Input: dimensioned drawing with shaded views. Units: mm. Origin: part minimum x, y, z. A direction names the side the tool comes from. Round coordinates to 2 decimals unless told otherwise and drop trailing zeros. Write each loop counter-clockwise with the first axis right and the second up, starting at its lowest first coordinate (ties: lowest second). Pieces come first, ordered by that corner, then holes. Notation, with made-up numbers: M -39.75,79.5 L 8.25,79.5 A31 ccw 8.25,106.5 Z; hole C 38,41.5 d10. An arc over 180 degrees is marked long. Put each result on its own line as item: value. Start each with the question number.
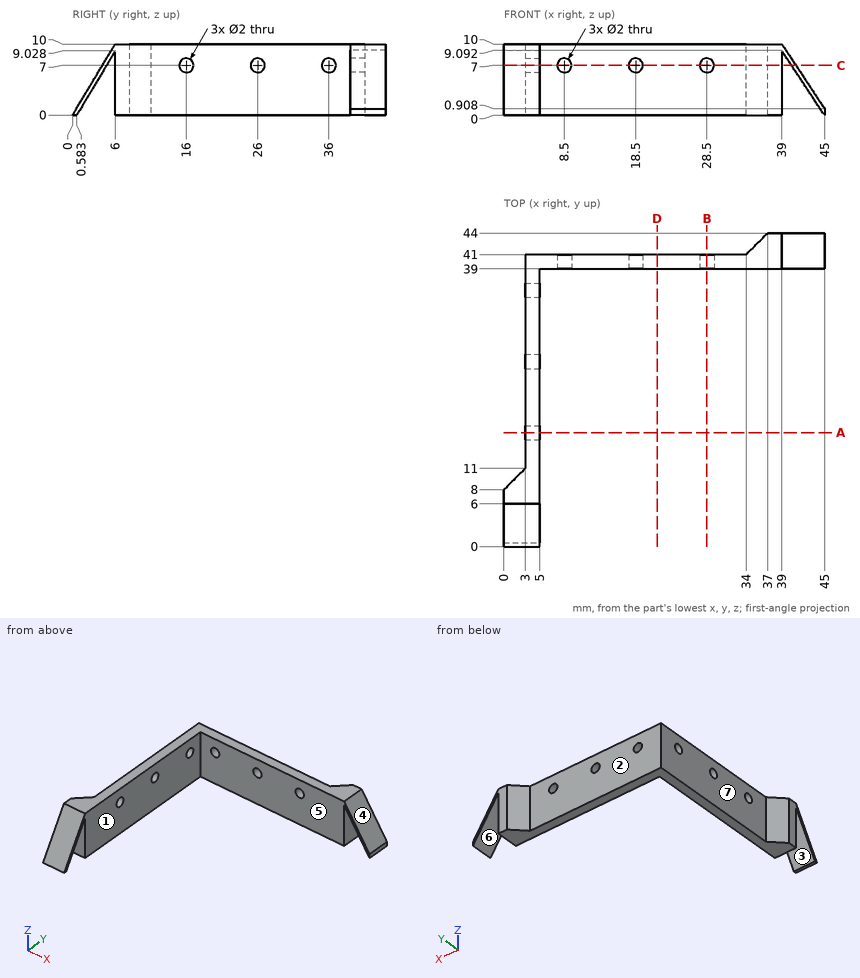
1) First-contact query: pin 1 (1.6 mm diameter, centred on x = 18.5, z = 7, fed in from +Y); pin 2 (3 mm diameter, centred on y = 27, z = 8.5, fed in from -X); pin 3 (1.5 mm diameter, centred on x = 23, z = 2.5, fed in from -Y); pin 4 (2.5 mm diameter, centred on y = 16, z = 7, fed in from +X). Flat tips, straight axial feed; report the tip coordinate or a pass-through.
2) Draft query along X for the marked faces 5, 6 and 7. Return one class per face: +X half, -X half, draft (parallel to the pull), parting line (faces both ways), or undercut.
3) Ray query, probe 1 along Z at (x, y) = (3.8, 16); probe 2 along Y at (x, z) = (14.5, 0.75); probe 3 along X at (y, z) = (8, 2.5). Return the intervals inside material, ascending.
4) Section A-A, the plane y = 16. Output: boundary loops of the cut face in (x, z), and give its area (3 significant figures).
5) Section D-D, the plane x = 21.5. Output: boundary loops of the cut face in (y, z), and give its area (3 significant figures).
6) Access query for the marked faces 1, 2, 3 and 4. Directions: +Z, -Z, +X, -X, +Y, -Y. A direction counts if a zero-diameter tool reaches every point of the face in a straight line with its end or side. Return the directions, or none.
7) Section B-B, the plane x = 28.5. Output: boundary loops of the cut face in (y, z), and give its area (3 significant figures).
8) Section C-C, the plane z = 7. Give the number of separate pieces and of enclosed holes in the cut face, and give its area (3 significant figures).
Solved:
1. pin 1: passes through
1. pin 2: stops at x = 3
1. pin 3: stops at y = 39
1. pin 4: stops at x = 5
2. face 5: draft
2. face 6: undercut
2. face 7: -X half
3. probe 1: z = 0 to 6, 8 to 10
3. probe 2: y = 39 to 41
3. probe 3: x = 0 to 5
4. outline: M 3,0 L 5,0 L 5,6 L 3,6 Z; M 3,8 L 5,8 L 5,10 L 3,10 Z
4. area: 16.0 mm2
5. outline: M 39,0 L 41,0 L 41,10 L 39,10 Z
5. area: 20.0 mm2
6. face 1: +Z, -Z, +X, -Y
6. face 2: +Z, -Z, -X, +Y
6. face 3: -Z, +X, -X
6. face 4: +Z, +X, +Y, -Y
7. outline: M 39,0 L 41,0 L 41,6 L 39,6 Z; M 39,8 L 41,8 L 41,10 L 39,10 Z
7. area: 16.0 mm2
8. separate pieces: 9
8. enclosed holes: 0
8. area: 141 mm2
